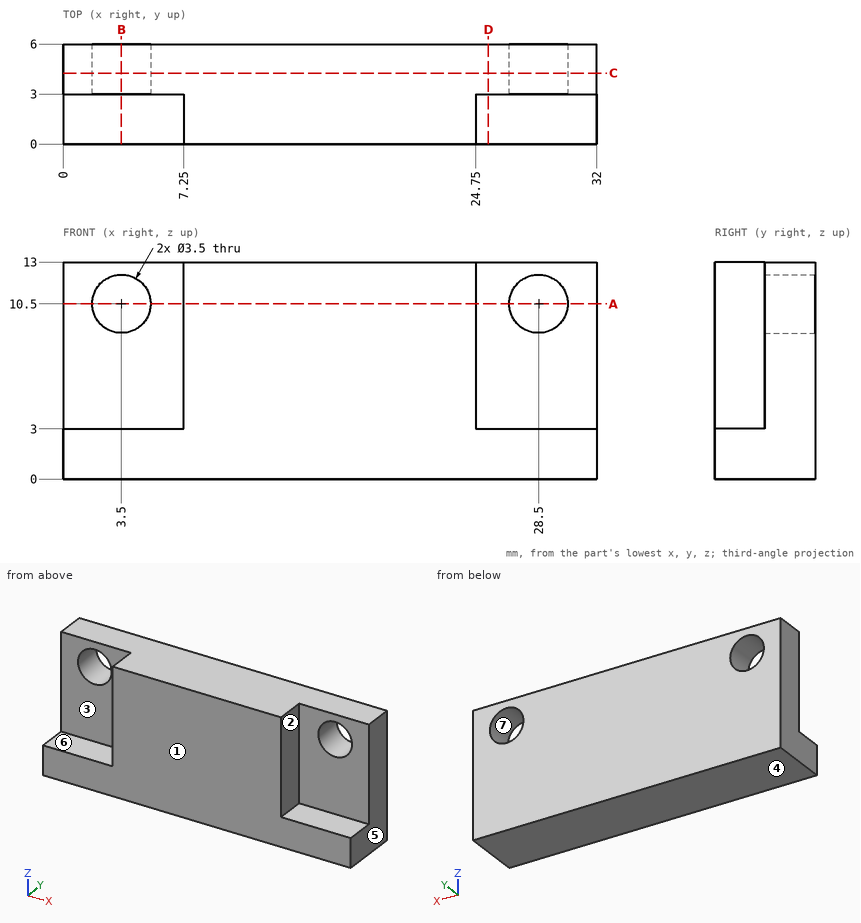
Here's the drawing with two shaded views (mm, measured from the low corner). I have some questions. A direction names the side the tool comes from. Round coordinates to 2 decimals unless told otherwise and drop trailing zeros. Write each loop counter-clockwise with the first axis right and the second up, starting at its lowest first coordinate (ties: lowest second). Pieces come first, ordered by that corner, then holes. Notation, with made-up numbers: M 45,16 L 101,16 A25 ccw 101,31 Z; hole C 0,-28.5 d3. An arc over 180 degrees is marked long. Answer in a Markdown table with one row per item. Add a question column.
Q1. If we mould it in two halves opening along Z, with no side actions, what happens to the marked faces 4, 5, 6 and 7? For each: +Z half, -Z half, draft (parallel to the pull), parting line (faces both ways), or undercut.
Q2. Imagine slicing it at A-A (z = 10.5). Please give me the cut outline in (x, y).
Q3. On a 3-axis mill with a long thin cutter (end or side, diameter ignored), from which of +Z, -Z, +X, -X, +Y, -Y can I reach the whole of each face in a straight line? I mean the marked faces 1, 2 and 3. Say none if no direction works.
Q4. Imagine slicing it at B-B (x = 3.5). Please give me the cut outline in (y, z), then the cut area to 3 significant figures.
Q5. Imagine slicing it at C-C (y = 4.25). Please give me the cut outline in (x, z).
Q6. Imagine slicing it at D-D (x = 25.5). Please give me the cut outline in (y, z).
Q7. Will these pins go through, and if not, where does the flat tip stop? pin 1 Ø2.5 at (y, z) = (1, 9.5) entering from -X; pin 2 Ø5.5 at (x, z) = (3.5, 10.5) entering from -Y; pin 3 Ø1 at (x, z) = (21.5, 3.5) entering from -Y; pin 4 Ø2.5 at (y, z) = (1.5, 10) entering from +X.
Q8. If I drill on line 1 (X direction, y = 4.5, z = 10.5); line 2 (Z direction, x = 3.5, y = 5); line 3 (X direction, y = 3.05, z = 9.25), over which ranges is the centre line in solid material (lowest first)? Write a range as from..to.
Values:
| question | item | result |
|---|---|---|
| 1 | face 4 | -Z half |
| 1 | face 5 | draft |
| 1 | face 6 | +Z half |
| 1 | face 7 | undercut |
| 2 | outline | M 0,3 L 1.75,3 L 1.75,6 L 0,6 Z; M 5.25,3 L 7.25,3 L 7.25,0 L 24.75,0 L 24.75,3 L 26.75,3 L 26.75,6 L 5.25,6 Z; M 30.25,3 L 32,3 L 32,6 L 30.25,6 Z |
| 3 | face 1 | +Z, -Z, +X, -X, -Y |
| 3 | face 2 | +Z, +X, -Y |
| 3 | face 3 | +Z, -X, -Y |
| 4 | outline | M 0,0 L 6,0 L 6,8.75 L 3,8.75 L 3,3 L 0,3 Z; M 3,12.25 L 6,12.25 L 6,13 L 3,13 Z |
| 4 | area | 37.5 mm^2 |
| 5 | outline | M 0,0 L 32,0 L 32,13 L 0,13 Z; hole C 3.5,10.5 d3.5; hole C 28.5,10.5 d3.5 |
| 6 | outline | M 0,0 L 6,0 L 6,13 L 3,13 L 3,3 L 0,3 Z |
| 7 | pin 1 | x = 7.25 |
| 7 | pin 2 | y = 3 |
| 7 | pin 3 | y = 0 |
| 7 | pin 4 | x = 24.75 |
| 8 | line 1 | 0..1.75, 5.25..26.75, 30.25..32 |
| 8 | line 2 | 0..8.75, 12.25..13 |
| 8 | line 3 | 0..2.28, 4.72..27.28, 29.72..32 |
